Read the model definition and answer for the solid it produces. Units are mm, in the model's axes. A direction names the side the tool comes from. Round coordinates to 2 decimals unless told otherwise and drop trailing zeros. Loops run counter-clockwise (first coordinate to the right, second up) from the corner with the lowest first, then second, coordinate; pieces in that order, holes last. Notation, with made-up numbers: M -9.5,-8 L 48.5,-8 A20 ccw 48.5,7 Z; hole C 62.25,-25 d2. An arc over 180 degrees is marked long. Write each question's results on one line, items separated by ' | '.
```python
from build123d import *

# Parameters (mm, degrees)
SKETCH1_R           = 33.3
BOSS_EXTRUDE1_DEPTH = 20
CIRPATTERN1_COUNT   = 3
CUT_EXTRUDE1_DEPTH  = 13
CUT_EXTRUDE3_REACH  = 53.164
SKETCH6_R           = 9.525
CUT_EXTRUDE4_START  = -1
SKETCH6_4_R         = 10.5
SKETCH6_4_R_2       = 9.525
CUT_EXTRUDE4_DEPTH  = 1
SKETCH7_R           = 0.8
SKETCH7_R_2         = 1.25
CUT_EXTRUDE5_DEPTH  = 52.164245328
SKETCH8_W           = 20.5
SKETCH8_H           = 25
CUT_EXTRUDE6_DEPTH  = 3.15
CUT_EXTRUDE7_REACH  = 52.017
SKETCH9_W           = 20.5
SKETCH9_H           = 20


with BuildPart() as part:
    # Sketch1 → Boss-Extrude1 (new body)
    with BuildSketch(Plane(origin=(0, 0, 0), x_dir=(1, 0, 0), z_dir=(0, 1, 0))):
        with Locations(Location((0, 0, 0), (0, 0, 270))):
            Circle(SKETCH1_R)
    extrude(amount=BOSS_EXTRUDE1_DEPTH)

    # Sketch3 → Cut-Revolve7 (revolve, cut)
    with BuildSketch(Plane.XZ):
        with BuildLine():
            Line((2.5019, 18), (-2.5019, 18))
            ThreePointArc((-2.5019, 18), (0, 15.4981), (2.5019, 18))
        make_face()
    cut_revolve7 = revolve(axis=Axis((3.292813159, 0, 18), (-1, 0, 0)), mode=Mode.SUBTRACT)

    # CirPattern1: Cut-Revolve7 ×3 about axis
    cirpattern1_axis = Axis((0, 0, 0), (0, 1, 0))
    for i in range(1, CIRPATTERN1_COUNT):
        add(cut_revolve7.rotate(cirpattern1_axis, i * 360 / CIRPATTERN1_COUNT), mode=Mode.SUBTRACT)

    # Sketch5 → Cut-Extrude1 (cut)
    with BuildSketch(Plane.XZ):
        with BuildLine():
            Line((9.525, -14), (9.525, 0))
            ThreePointArc((9.525, 0), (0, 9.525), (-9.525, 0))
            Line((-9.525, 0), (-9.525, -14))
            Line((-9.525, -14), (-21.202606522, -25.677606522))
            ThreePointArc((-21.202606522, -25.677606522), (0, -33.3), (21.202606522, -25.677606522))
            Line((21.202606522, -25.677606522), (9.525, -14))
        make_face()
    extrude(amount=-CUT_EXTRUDE1_DEPTH, mode=Mode.SUBTRACT)

    # Sketch6 → Cut-Extrude3 (cut, up to next)
    with BuildSketch(Plane(origin=(0, 20, 0), x_dir=(1, 0, 0), z_dir=(0, 1, 0)), mode=Mode.PRIVATE) as cut_extrude3_sk1:
        Circle(SKETCH6_R)
    cut_extrude3_tool1 = extrude(cut_extrude3_sk1.sketch, amount=-CUT_EXTRUDE3_REACH, mode=Mode.PRIVATE) & part.part
    add(cut_extrude3_tool1.solids().sort_by_distance((0, 20, 0))[0], mode=Mode.SUBTRACT)

    # Sketch6_4 → Cut-Extrude4 (cut)
    with BuildSketch(Plane(origin=(0, 20, 0), x_dir=(1, 0, 0), z_dir=(0, 1, 0)).offset(CUT_EXTRUDE4_START)):
        with Locations(Location((0, 0, 0), (0, 0, 270))):
            Circle(SKETCH6_4_R)
        Circle(SKETCH6_4_R_2, mode=Mode.SUBTRACT)
    extrude(amount=CUT_EXTRUDE4_DEPTH, mode=Mode.SUBTRACT)

    # Sketch7 → Cut-Extrude5 (cut, through all)
    with BuildSketch(Plane(origin=(0, 20, 0), x_dir=(1, 0, 0), z_dir=(0, 1, 0))):
        with Locations(Location((-7.03, 14.5, 0), (0, 0, 270))):
            Circle(SKETCH7_R)
        with Locations(Location((7.03, 14.5, 0), (0, 0, 270))):
            Circle(SKETCH7_R)
        with Locations(Location((1.13, 15.4, 0), (0, 0, 270))):
            Circle(SKETCH7_R_2)
    extrude(amount=-CUT_EXTRUDE5_DEPTH, mode=Mode.SUBTRACT)

    # Sketch8 → Cut-Extrude6 (cut)
    with BuildSketch(Plane(origin=(0, 20, 0), x_dir=(1, 0, 0), z_dir=(0, 1, 0))):
        with Locations((0, 24.1)):
            Rectangle(SKETCH8_W, SKETCH8_H)
    extrude(amount=-CUT_EXTRUDE6_DEPTH, mode=Mode.SUBTRACT)

    # Sketch9 → Cut-Extrude7 (cut, up to next)
    with BuildSketch(Plane(origin=(0, 16.85, 0), x_dir=(1, 0, 0), z_dir=(0, 1, 0)), mode=Mode.PRIVATE) as cut_extrude7_sk1:
        with Locations((0, 28.3)):
            Rectangle(SKETCH9_W, SKETCH9_H)
    cut_extrude7_tool1 = extrude(cut_extrude7_sk1.sketch, amount=-CUT_EXTRUDE7_REACH, mode=Mode.PRIVATE) & part.part
    add(cut_extrude7_tool1.solids().sort_by_distance((0, 16.85, -28.3))[0], mode=Mode.SUBTRACT)


solid = part.part
```
1. Find section A-A, the plane x = 1.13. Give the vertices of the cut face in (y, z), then the cut area to 3 significant figures.
Completed:
outline: M 0,9.46 L 19,9.46 L 19,10.44 L 20,10.44 L 20,33.28 L 0,33.28 L 0,20.23 A2.23 cw 0,15.77 Z; M 13,-18.3 L 16.85,-18.3 L 16.85,-16.65 L 13,-16.65 Z; M 13,-14.15 L 16.85,-14.15 L 16.85,-11.6 L 20,-11.6 L 20,-10.44 L 19,-10.44 L 19,-9.46 L 13,-9.46 Z | area: 498 mm2
2. Which of the six approach directions +Z, -Z, +X, -X, +Y, -Y give full straight-line access (tool end or side, diameter ignored) to faces 4 (the face through (-10.25, 17, -24)), 5 (the face through (-15.282, 6.409, -19.757)), 6 (the face through (-9, 19, 5))?
Completed:
face 4: -Z, +Y | face 5: -Z, -Y | face 6: +Y
3. Find the intervals of material crossed by L1, parallel to X at y = 13.9, z = -14.5; L2, parallel to X at y = 19.7, z = 0; L3, parallel to Y at x = 11, z = -16.5, in increasing order.
Completed:
L1: x = -29.98 to -7.83, -6.23 to 0.26, 2 to 6.23, 7.83 to 29.98 | L2: x = -33.3 to -10.5, 10.5 to 33.3 | L3: y = 13 to 20
4. Find section C-C, the plane y = 14.75. Give the vertices of the cut face in (x, z) (3 decimals), then the cut area to 3 significant figures.
Completed:
outline: M -10.25,-31.683 L -10.25,-18.3 L 10.25,-18.3 L 10.25,-31.683 A33.3 ccw long Z; hole C 0,0 d19.05; hole C -7.03,-14.5 d1.6; hole C 1.13,-15.4 d2.5; hole C 7.03,-14.5 d1.6 | area: 2,890 mm2
5. Determine the mould class of faces 1 (the face through (0, 0, 10)), 2 (the face through (-7.52, 14.95, -15.13)), 3 (the face through (0, 15, -18.3)) for opening direction Z: released by +Z, released by -Z, zero draft, split by the parting line, or undercut.
Completed:
face 1: zero draft | face 2: undercut | face 3: released by -Z
6. Given P1, Ø1.2, axis at x = 1, y = 14, coming from the -Z side; P2, Ø1, axis at y = 7.5, z = 24.5, coming from the -X side; P3, Ø2, axis at y = 16, z = -18, coming from the +X side, each flat-ended and moving along its own axis, determine where each tip first touches the part or whether it passes through.
Completed:
P1: stops at z = -18.3 | P2: stops at x = -23.08 | P3: stops at x = 28.63
7. Find section B-B, the plane z = -4.5. Give the vertices of the cut face in (x, y) (3 decimals), then the cut area to 3 significant figures.
Completed:
outline: M -32.995,0 L -9.525,0 L -9.525,13 L -8.395,13 L -8.395,19 L -9.487,19 L -9.487,20 L -32.995,20 Z; M 8.395,13 L 9.525,13 L 9.525,0 L 32.995,0 L 32.995,20 L 9.487,20 L 9.487,19 L 8.395,19 Z | area: 952 mm2
8. Find section D-D, the plane y = 8.75. Give the vertices of the cut face in (x, z) (3 decimals), then the cut area to 3 significant figures.
Completed:
outline: M -21.203,-25.678 L -9.525,-14 L -9.525,0 A9.525 cw 9.525,0 L 9.525,-14 L 21.203,-25.678 A33.3 ccw long Z | area: 2,490 mm2
